from build123d import *
from build123d import SkipClean  # not in build123d's __all__

# Parameters (mm, degrees)
F0_R      = 63.5
F1_DEPTH  = 25.4
F2_R      = 19.05
F3_DEPTH  = 25.401
F4_R      = 6.35
F5_DEPTH  = 25.4
F6_R      = 9.525
F7_DEPTH  = 6.35
F8_W      = 50.8
F8_H      = 50.8
F9_DEPTH  = 95.25
F10_R     = 19.05
F11_DEPTH = 88.9
F12_R     = 11.4435821265
F12_R_2   = 8.6754099319
F12_R_3   = 6.35
F13_DEPTH = 25.4
F14_R     = 12.7
F15_DEPTH = 25.4
F16_R     = 9.525
F17_DEPTH = 25.4
F18_R     = 11.9876896331
F18_R_2   = 9.525
F19_DEPTH = 9.525


# Not quite as in the source:
# - after a boolean that leaves OpenCascade's solid faulty, fix() repairs it


with BuildPart() as f1:
    # F0 (on Front) → F1 (new body)
    with BuildSketch(Plane.XZ):
        Circle(F0_R)
    extrude(amount=F1_DEPTH)

    # F2 (on face) → F3 (cut, through all)
    with BuildSketch(Plane.XZ.offset(25.4)):
        Circle(F2_R)
    extrude(amount=-F3_DEPTH, mode=Mode.SUBTRACT)

    # F4 (on face) → F5 (cut)
    with BuildSketch(Plane.XZ.offset(25.4)):
        with Locations((50.8, 0)):
            Circle(F4_R)
    extrude(amount=-F5_DEPTH, mode=Mode.SUBTRACT)

    # F6 (on face) → F7 (cut)
    with BuildSketch(Plane.XZ.offset(25.4)):
        with Locations((50.8, 0)):
            Circle(F6_R)
    extrude(amount=-F7_DEPTH, mode=Mode.SUBTRACT)

    # F8 (on face) → F9 (join)
    with BuildSketch(Plane(origin=(0, 0, 0), x_dir=(-1, 0, 0), z_dir=(0, 1, 0))):
        Rectangle(F8_W, F8_H)
    extrude(amount=F9_DEPTH)

    # F10 (on face) → F11 (cut)
    with BuildSketch(Plane(origin=(0, 95.25, 0), x_dir=(-1, 0, 0), z_dir=(0, 1, 0))):
        Circle(F10_R)
    extrude(amount=-F11_DEPTH, mode=Mode.SUBTRACT)

    # F12 (on face) → F13 (join)
    with BuildSketch(Plane(origin=(0, 0, 0), x_dir=(-1, 0, 0), z_dir=(0, 1, 0))):
        with Locations((-50.8, 0)):
            Circle(F12_R)
        with Locations((-50.8, 0)):
            Circle(F12_R_2, mode=Mode.SUBTRACT)
        with Locations((-50.8, 0)):
            Circle(F12_R_2)
        with Locations((-50.8, 0)):
            Circle(F12_R_3, mode=Mode.SUBTRACT)
    with SkipClean():  # cleaning this boolean's faces spoils the solid; the shape is the same uncleaned
        extrude(amount=F13_DEPTH)

    # F14 (on face) → F15 (join)
    with BuildSketch(Plane.XY.offset(25.4)):
        with Locations((0, 33.4604047239)):
            Circle(F14_R)
    extrude(amount=F15_DEPTH)

    add(f1.part.fix(), mode=Mode.REPLACE)

    # F16 (on face) → F17 (cut)
    with BuildSketch(Plane.XY.offset(50.8)):
        with Locations((0, 33.4604047239)):
            Circle(F16_R)
    extrude(amount=-F17_DEPTH, mode=Mode.SUBTRACT)

    add(f1.part.fix(), mode=Mode.REPLACE)

    # F18 (on face) → F19 (join)
    with BuildSketch(Plane.XZ.offset(25.4)):
        with Locations((50.8, 0)):
            Circle(F18_R)
        with Locations((50.8, 0)):
            Circle(F18_R_2, mode=Mode.SUBTRACT)
    extrude(amount=F19_DEPTH)


solid = f1.part
Read the model definition and answer for the solid it produces. Units are mm, in the model's axes. A direction names the side the tool comes from. Give positions to 0.01 mm unless a question says otherwise; leave off trailing zeros. Write each loop counter-clockwise with the first axis right and the second up, starting at its lowest first coordinate (ties: lowest second). Pieces come first, ordered by that corner, then holes. Notation, with made-up numbers: (82.25, 18.25) -> (128.25, 18.25) arc R5 cw to (128.25, 27.25) -> close; hole circle Ø9 at (-21, -28). An arc over 180 degrees is marked (long way). Answer as a JSON object with one key per item and string values. Group by question number.
1) The mould has two halves that part along Y. Classify faces 6 (the flat face through (0, 47, 25.4)), 7 (the flat face through (0, 6.35, 0)), 8 (the cylindrical face through (39.885, 12.522, 3.437)): +Y half, -Y half, draft (parallel to the pull), parting line (faces both ways), or undercut.
2) Find section D-D (x = 0). Write down the section's boundary in (y, z).
3) Find section A-A (y = 16.5). Write down the section's boundary in (x, z).
4) Find section C-C (x = 50.8). Write down the section's boundary in (y, z) (3 decimals), and give its area (3 significant figures).
5) A tool of negligible diameter and unlimited length cuts with its end or side. For faces 1 (the flat face through (0, 34, 25.4)), 2 (the cylindrical face through (62.234, -30.096, 3.601)), 3 (the flat face through (0, 47, -25.4)), 4 (the flat face through (2, 43, 50.8)), 5 (the flat face through (-25.4, 47, 0)), from which of +Z, -Z, +X, -X, +Y, -Y can it reach the whole face along a straight path? Write none if from no direction.
6) Consider L1, parallel to Z at x = 50.8, y = 6.5; L2, parallel to Z at x = 50.8, y = -29.5 (3 decimals); L3, parallel to Z at x = 19.5, y = 45. Determine where each line is inside the solid, lowest interval first. Write a range as from..to.
7) Each of these flat-tipped pins is pushed along its axis until it touches: P1, Ø10, axis at x = 20, z = 13.5, coming from the -Y side; P2, Ø10, axis at x = -44, z = -33.5, coming from the +Y side; P3, Ø11.5, axis at x = 49.5, z = 1, coming from the +Y side. Where does it stop, or does it pass through?
Values follow:
{
 "1": {"face 6": "undercut", "face 7": "+Y half", "face 8": "draft"},
 "2": {"outline": "(-25.4, -63.5) -> (0, -63.5) -> (0, -25.4) -> (95.25, -25.4) -> (95.25, -19.05) -> (6.35, -19.05) -> (6.35, 19.05) -> (95.25, 19.05) -> (95.25, 25.4) -> (46.16, 25.4) -> (46.16, 50.8) -> (42.99, 50.8) -> (42.99, 25.4) -> (23.94, 25.4) -> (23.94, 50.8) -> (20.76, 50.8) -> (20.76, 25.4) -> (0, 25.4) -> (0, 63.5) -> (-25.4, 63.5) -> (-25.4, 19.05) -> (0, 19.05) -> (0, -19.05) -> (-25.4, -19.05) -> close"},
 "3": {"outline": "(-25.4, -25.4) -> (25.4, -25.4) -> (25.4, 25.4) -> (-25.4, 25.4) -> close; circle Ø22.89 at (50.8, 0); hole circle Ø38.1 at (0, 0); hole circle Ø12.7 at (50.8, 0)"},
 "4": {"outline": "(-34.925, -11.988) -> (-25.4, -11.988) -> (-25.4, -38.1) -> (0, -38.1) -> (0, -11.444) -> (25.4, -11.444) -> (25.4, -6.35) -> (-19.05, -6.35) -> (-19.05, -9.525) -> (-34.925, -9.525) -> close; (-34.925, 9.525) -> (-19.05, 9.525) -> (-19.05, 6.35) -> (25.4, 6.35) -> (25.4, 11.444) -> (0, 11.444) -> (0, 38.1) -> (-25.4, 38.1) -> (-25.4, 11.988) -> (-34.925, 11.988) -> close", "area": "1,880 mm2"},
 "5": {"face 1": "+Z", "face 2": "-Y", "face 3": "-Z, +X, -X, +Y", "face 4": "+Z, +X, -X, +Y", "face 5": "+Z, -Z, -X, +Y"},
 "6": {"L1": "z = -11.44..-6.35, 6.35..11.44", "L2": "z = -11.988..-9.525, 9.525..11.988", "L3": "z = -25.4..25.4"},
 "7": {"P1": "stops at y = -25.4", "P2": "stops at y = 0", "P3": "stops at y = 25.4"}
}
